Autodesk Inventor part; units mm, degrees
ref_plane "MSC_PF1" through (0, 0, 0) normal (1, 0, 0) x (0, 1, 0)
ref_plane "MSC_PT1" through (0, 0, 0) normal (0, 0, -1) x (-1, 0, 0)
ref_plane "YZ Plane" through (0, 0, 0) normal (1, 0, 0) x (0, 1, 0)
sketch "Sketch1" plane through (0, 0, 0) normal (0, 1, 0) x (-1, 0, 0)
  point P0 (0, 0)
sketch "Sketch2" plane through (0, 0, 0) normal (0, 1, 0) x (-1, 0, 0)
  line L0 (-4, -25) -> (0, -25)
  line L1 (-4, -4.4) -> (-4, -25)
  line L2 (-8, -0.4) -> (-4, -4.4)
  line L3 (-8, 0) -> (-8, -0.4)
  line L4 (0, 0) -> (-8, 0)
  line L5 (0, -25) -> (0, 0)
  line L6 (0, -25) -> (0, 0)
  line L7 (0, -30) -> (0, 5)
  line L8 (1.6, 0) -> (-9.6, 0)
  dimension "d3" = 8
  dimension "d5" = 4
  dimension "d7" = 25
  dimension "ParC" = 0.4
  dimension "d22" = 0
  dimension "d23" = 0
  dimension "d43" = 45
revolve "Revolution1" add sketch "Sketch2" angle 360 about axis through (0, 0, -25) along (0, 0, -1)
sketch "Sketch3" plane through (0, 0, 0) normal (0, 0, 1) x (1, 0, 0)
  line L0 (-2.5, 1.4434) -> (-2.5, -1.4434)
  line L1 (0, 2.8868) -> (-2.5, 1.4434)
  line L2 (2.5, 1.4434) -> (0, 2.8868)
  line L3 (2.5, -1.4434) -> (2.5, 1.4434)
  line L4 (0, -2.8868) -> (2.5, -1.4434)
  line L5 (-2.5, -1.4434) -> (0, -2.8868)
  circle A0 centre (0, 0) radius 2.5 construction
  circle A1 centre (0, 0) radius 4 construction
  dimension "d11" = 5
  dimension "d13" = 120
  dimension "d15" = 120
extrude "Extrusion1" cut sketch "Sketch3" against normal blind 3.5
fillet "Fillet1" radius 0.5 1 edges at (-4, 0, -4.4)
chamfer "Chamfer1" distance 0.625 angle 45 1 edges at (-4, 0, -25) measured on face at (-0.9596, 3.8832, -18.2024)
thread "Thread1"
ref_plane "MSC_PF1" through (0, 0, 0) normal (1, 0, 0) x (0, 1, 0)
ref_plane "MSC_PT1" through (0, 0, 0) normal (0, 0, -1) x (-1, 0, 0)
equation "\"d3\" = 0.5 * dk"
equation "\"d5\" = 0.5 * NND"
equation "\"d7\" = NLG"
equation "\"d43\" = 0.5 * ang"
equation "\"d18\" = r"
equation "\"d19\" = 0.5 * PTC"
equation "\"d39\" = 0.5 * PTC"
equation "\"d11\" = ParS"
equation "\"d16\" = ParT"
equation "\"NND\" = 8"
equation "\"PTC\" = 1.25"
equation "\"dk\" = 16"
equation "\"ParK\" = 4.4"
equation "\"ParS\" = 5"
equation "\"ParT\" = 3.5"
equation "\"r\" = 0.5"
equation "\"NLG\" = 25"
equation "\"ang\" = 90deg"
equation "\"THREADDIA\" = NND"
properties part number "ISO 10642 - M8x25" material "Steel, Mild"
The model under review builds one solid part; all positions refer to its coordinate system, in mm. A direction names the side the tool comes from. Give positions to 0.01 mm unless a question says otherwise; leave off trailing zeros. Loops run counter-clockwise (first coordinate to the right, second up) from the corner with the lowest first, then second, coordinate; pieces in that order, holes last. Notation, with made-up numbers: (84.25, 84.5) -> (139.25, 84.5) arc R36 cw to (139.25, 119.5) -> close; hole circle Ø10 at (21.25, 5). An arc over 180 degrees is marked (long way). Use CSV: the item, a comma, the result in double quotes.
1. For P1, Ø0.9, axis at y = -0.5, z = -1, coming from the -X side; P2, Ø1, axis at y = -1.5, z = -8.5, coming from the -X side; P3, Ø1, axis at y = -3.5, z = -6, coming from the +X side, all flat-tipped, find the tip position at first contact; note any pin that passes through.
Result:
P1,"stops at x = -7.83"
P2,"stops at x = -3.87"
P3,"stops at x = 2.65"
2. The part is to be moulded in two halves that separate along Y. For faces 4 (the face through (2.025, -3.892, -4.013)), 5 (the face through (-2.5, 0, -2)), 6 (the face through (-1.233, 2.175, -1.726)), 7 (the face through (0, 0, -25)), say which applies: +Y half, -Y half, draft (parallel to the pull), parting line (faces both ways), or undercut.
Result:
face 4,"parting line"
face 5,"undercut"
face 6,"undercut"
face 7,"draft"
3. To check wall thickness, follow probe 1 along X at (y, z) = (-0.5, -1.75); probe 2 along Z at (x, y) = (-2.75, -3.5); probe 3 along Y at (x, z) = (2, -12.75). State the ranges of each line that lie inside material, in increasing order. Write a range as from..to.
Result:
probe 1,"x = -6.63..-2.5, 2.5..6.63"
probe 2,"z = -3.95..0"
probe 3,"y = -3.46..3.46"
4. Machinability: for faces 1 (the face through (-0.867, 3.905, -14.629)), 2 (the face through (-2, -2, 0)), 3 (the face through (1.233, -2.175, -1.726)), which of the approach directions +Z, -Z, +X, -X, +Y, -Y give a long, thin tool a straight path to every point of the face, cutting with its end or side? Answer none if there is none.
Result:
face 1,"-Z"
face 2,"+Z, +X, -X, +Y, -Y"
face 3,"+Z"
5. Consider section A-A, the plane z = -16.75. Write out the cut boundary in (x, y), then the cut area to 3 significant figures.
Result:
outline,"circle Ø8 at (0, 0)"
area,"50.3 mm²"
